from build123d import *

# Parameters (mm, degrees)
F0_W     = 34.6
F0_H     = 17.5
F1_DEPTH = 38
F2_DEPTH = 23
F3_R     = 2.5
F4_DEPTH = 25.501001
F5_R     = 2


with BuildPart() as f1:
    # F0 (on Top) → F1 (new body)
    with BuildSketch(Plane.XY):
        with BuildLine():
            Line((36.600001, 21.500001), (-2.000001, 21.500001))
            ThreePointArc((-2.000001, 21.500001), (-3.414214, 20.914214), (-4.000001, 19.500001))
            Line((-4.000001, 19.500001), (-4.000001, -2.000001))
            ThreePointArc((-4.000001, -2.000001), (-3.414214, -3.414214), (-2.000001, -4.000001))
            Line((-2.000001, -4.000001), (36.600001, -4.000001))
            ThreePointArc((36.600001, -4.000001), (38.014214, -3.414214), (38.600001, -2.000001))
            Line((38.600001, -2.000001), (38.600001, 19.500001))
            ThreePointArc((38.600001, 19.500001), (38.014214, 20.914214), (36.600001, 21.500001))
        make_face()
        with Locations((17.3, 8.75)):
            Rectangle(F0_W, F0_H, mode=Mode.SUBTRACT)
        with Locations((17.3, 8.75)):
            Rectangle(F0_W, F0_H)
    extrude(amount=-F1_DEPTH)

    # F0 (on Top) → F2 (cut)
    with BuildSketch(Plane.XY):
        with Locations((17.3, 8.75)):
            Rectangle(F0_W, F0_H)
    extrude(amount=-F2_DEPTH, mode=Mode.SUBTRACT)

    # F3 (on face) → F4 (cut, through all)
    with BuildSketch(Plane.XZ.offset(4.000001)):
        with BuildLine():
            ThreePointArc((22.039303, -30.356017), (24.539303, -32.856017), (27.039303, -30.356017))
            ThreePointArc((27.039303, -30.356017), (24.539303, -27.856017), (22.039303, -30.356017))
        make_face()
        with Locations((9.539303, -30.356017)):
            Circle(F3_R)
    extrude(amount=-F4_DEPTH, mode=Mode.SUBTRACT)

    # F5
    f5_edges = [f1.edges().sort_by_distance(p)[0] for p in [
        (17.3, 21.500001, -38),
    ]]
    fillet(f5_edges, radius=F5_R)


solid = f1.part
Input: part model. Units: mm. Frame: model coordinates. A direction names the side the tool comes from. Coordinates: 2 decimals unless noted, no trailing zeros. Loops run counter-clockwise (first coordinate to the right, second up) from the corner with the lowest first, then second, coordinate; pieces in that order, holes last. Notation, with made-up numbers: (17, -32.5) -> (23, -32.5) arc R20 cw to (23, 0.5) -> close; hole circle Ø1 at (0, 74). An arc over 180 degrees is marked (long way). Write each question's results on one line, items separated by ' | '. Start each with the question number.
Q1. Section A-A, the plane z = -13. Return the cut outline in (x, y).
Q2. Section B-B, the plane x = 25.5. Return the cut outline in (y, z), plus the area to 3 significant figures.
Q3. Pull-direction query (X, two-part tool) for faces 3 (the flat face through (17, 9, -23)), 4 (the cylindrical face through (-3.43, -3.4, -17.75)), 5 (the flat face through (17, 0, -11)), 6 (the cylindrical face through (17.03, 20.93, -37.4)); classes: released by +X, released by -X, zero draft, split by the parting line, or undercut.
Q4. Reachability of faces 1 (the flat face through (17, -4, -18)), 2 (the flat face through (17, 17.5, -11)) from +Z, -Z, +X, -X, +Y, -Y: full face, straight path, thin tool, end or side. Return the list, or none.
Q5. Ray query, line 1 (Y direction, x = 2.5, z = -17); line 2 (X direction, y = 9, z = -4); line 3 (Z direction, x = 17.5, y = 6). Return the intervals inside material, ascending. Write a range as from..to.
Q6. Section C-C, the plane y = 4.75. Return the cut outline in (x, z).
Q7. Section D-D, the plane x = 16. Return the cut outline in (y, z), plus the area to 3 significant figures.
Found:
1) outline: (-4, -2) arc R2 ccw to (-2, -4) -> (36.6, -4) arc R2 ccw to (38.6, -2) -> (38.6, 19.5) arc R2 ccw to (36.6, 21.5) -> (-2, 21.5) arc R2 ccw to (-4, 19.5) -> close; hole (0, 0) -> (34.6, 0) -> (34.6, 17.5) -> (0, 17.5) -> close
2) outline: (-4, -36) arc R2 ccw to (-2, -38) -> (19.5, -38) arc R2 ccw to (21.5, -36) -> (21.5, -32.66) -> (-4, -32.66) -> close; (-4, -28.05) -> (21.5, -28.05) -> (21.5, 0) -> (17.5, 0) -> (17.5, -23) -> (0, -23) -> (0, 0) -> (-4, 0) -> close | area: 447 mm2
3) face 3: undercut | face 4: released by -X | face 5: undercut | face 6: zero draft
4) face 1: +Z, -Z, +X, -X, -Y | face 2: +Z
5) line 1: -4..0, 17.5..21.5 | line 2: -4..0, 34.6..38.6 | line 3: -38..-23
6) outline: (-4, -36) arc R2 ccw to (-2, -38) -> (36.6, -38) arc R2 ccw to (38.6, -36) -> (38.6, 0) -> (34.6, 0) -> (34.6, -23) -> (0, -23) -> (0, 0) -> (-4, 0) -> close; hole circle Ø5 at (9.54, -30.36); hole circle Ø5 at (24.54, -30.36)
7) outline: (-4, -36) arc R2 ccw to (-2, -38) -> (19.5, -38) arc R2 ccw to (21.5, -36) -> (21.5, 0) -> (17.5, 0) -> (17.5, -23) -> (0, -23) -> (0, 0) -> (-4, 0) -> close | area: 565 mm2
